Check sheet for the modelled part. Datum: model origin and axes. Units: mm. A direction names the side the tool comes from. Round coordinates to 2 decimals unless told otherwise and drop trailing zeros. Order: outer loops, then holes, each group sorted by start corner. A loop starts at its lowest first (then second) coordinate and runs counter-clockwise, first axis right, second up.
(1) Tool access check on faces 1 (the flat face through (-21, 32.1, 0)), 2 (the flat face through (1, 2, 0)). Record the directions out of +Z, -Z, +X, -X, +Y, -Y that give a thin tool (end or side, any length) a straight path to the whole face; none if there is none.
(2) Thickness scan on probe 1 along X at (y, z) = (6, 6) (3 decimals); probe 2 along Y at (x, z) = (-17, -9.5); probe 3 along Y at (x, z) = (-20.55, -10.5). Record the ranges inside material, lowest first.
(3) Sectioned sample at B-B, the plane y = 24.9. Enter the section's corners in (x, z) (3 decimals), and give its area (3 significant figures).
(4) Sectioned sample at D-D, the plane y = 13.5. Enter the section's corners in (x, z) (3 decimals).
(5) Sectioned sample at A-A, the plane z = 11. Enter the section's corners in (x, y) (3 decimals), and give its area (3 significant figures).
(6) Sectioned sample at C-C, the plane z = -11. Enter the section's corners in (x, y) (3 decimals).
(7) Depth check by flat-ended pin: pin 1 (12 mm diameter, centred on x = 5, y = 6, fed in from +Z); pin 2 (5 mm diameter, centred on y = 24.9, z = -10.5, fed in from +X); pin 3 (19 mm diameter, centred on x = -8, z = 2, fed in from +Y). Enter the tip coordinate at first touch or a pass-through.
(8) Mould release check, pull along X, two halves, no side actions. Record for faces 3 (the flat face through (-21.875, 16, 0)), 4 (the flat face through (21.875, 1, 0)), 5 (the flat face through (-6.6, 1.7, -19)), 6 (the cylindrical face through (18.41, 0.99, -11.95)): released by +X, released by -X, zero draft, split by the parting line, or undercut.
```python
from build123d import *

# Parameters (mm, degrees)
SKETCH1_W  = 43.75
SKETCH1_H  = 38
SKETCH1_R  = 3.15
BASE_DEPTH = 2
SKETCH2_W  = 38
SKETCH2_H  = 32.1
SKETCH2_R  = 3.2
TAB_DEPTH  = 2


with BuildPart() as part:
    # Sketch1 → Base (new body)
    with BuildSketch(Plane(origin=(0, 0, 0), x_dir=(1, 0, 0), z_dir=(0, 1, 0))):
        Rectangle(SKETCH1_W, SKETCH1_H)
        with Locations((15.405, 11)):
            Circle(SKETCH1_R, mode=Mode.SUBTRACT)
        with Locations((15.405, -11)):
            Circle(SKETCH1_R, mode=Mode.SUBTRACT)
    extrude(amount=BASE_DEPTH)

    # Sketch2 → Tab (add)
    with BuildSketch(Plane.ZY.offset(21.875)):
        with Locations((0, 16.05)):
            Rectangle(SKETCH2_W, SKETCH2_H)
        with Locations((-10.5, 24.9)):
            Circle(SKETCH2_R, mode=Mode.SUBTRACT)
    extrude(amount=-TAB_DEPTH)


solid = part.part
```
Derived:
1. face 1: +Z, -Z, +X, -X, +Y
1. face 2: +Z, -Z, +X, +Y
2. probe 1: x = -21.875 to -19.875
2. probe 2: y = 0 to 2
2. probe 3: y = 0 to 21.7, 28.1 to 32.1
3. outline: (-21.875, -19) - (-19.875, -19) - (-19.875, -13.7) - (-21.875, -13.7) - close; (-21.875, -7.3) - (-19.875, -7.3) - (-19.875, 19) - (-21.875, 19) - close
3. area: 63.2 mm2
4. outline: (-21.875, -19) - (-19.875, -19) - (-19.875, 19) - (-21.875, 19) - close
5. outline: (-21.875, 0) - (12.255, 0) - (12.255, 2) - (-19.875, 2) - (-19.875, 32.1) - (-21.875, 32.1) - close; (18.555, 0) - (21.875, 0) - (21.875, 2) - (18.555, 2) - close
5. area: 135 mm2
6. outline: (-21.875, 0) - (12.255, 0) - (12.255, 2) - (-19.875, 2) - (-19.875, 21.739) - (-21.875, 21.739) - close; (-21.875, 28.061) - (-19.875, 28.061) - (-19.875, 32.1) - (-21.875, 32.1) - close; (18.555, 0) - (21.875, 0) - (21.875, 2) - (18.555, 2) - close
7. pin 1: stops at z = 19
7. pin 2: passes through
7. pin 3: stops at y = 2
8. face 3: released by -X
8. face 4: released by +X
8. face 5: zero draft
8. face 6: undercut
